```python
from build123d import *

# Parameters (mm, degrees)
LINEAR_AUSTRAGEN_D_NN1_DEPTH    = 110
SKIZZE2_R                       = 2.5
SCHNITT_LINEAR_AUSTRAGEN1_DEPTH = 17
VERRUNDUNG1_R                   = 2


with BuildPart() as part:
    # Skizze1 → Linear-Austragen-Dünn1 (new body)
    with BuildSketch(Plane.XY):
        Polygon((0, 20), (0, 0), (20, 0), (20, 1.5), (1.5, 1.5), (1.5, 20), align=None)
    extrude(amount=-LINEAR_AUSTRAGEN_D_NN1_DEPTH)

    # Skizze2 → Schnitt-Linear austragen1 (cut)
    with BuildSketch(Plane.XZ):
        with Locations(Location((6.5, -27, 0), (0, 0, 270))):
            Circle(SKIZZE2_R)
    extrude(amount=-SCHNITT_LINEAR_AUSTRAGEN1_DEPTH, mode=Mode.SUBTRACT)

    # Verrundung1
    verrundung1_edges = [part.edges().sort_by_distance(p)[0] for p in [
        (0.75, 20, -110),
        (0.75, 20, 0),
        (20, 0.75, 0),
        (20, 0.75, -110),
    ]]
    fillet(verrundung1_edges, radius=VERRUNDUNG1_R)


solid = part.part
```
For this review, take the finished solid that the model builds, in its own axes (mm). A direction names the side the tool comes from. Give positions to 0.01 mm unless a question says otherwise; leave off trailing zeros. Write each loop counter-clockwise with the first axis right and the second up, starting at its lowest first coordinate (ties: lowest second). Pieces come first, ordered by that corner, then holes. Notation, with made-up numbers: M -29.5,44.25 L -4.5,44.25 A23 cw -4.5,67.25 Z; hole C -17.75,89 d4. An arc over 180 degrees is marked long. One line per item, written item: value.
1) For P1, Ø9, axis at y = 14, z = -54, coming from the +X side, flat-tipped, find the tip position at first contact; note if it passes through.
Results are:
P1: stops at x = 1.5
2) For line 1 (X direction, y = 0.6, z = -27); line 2 (X direction, y = 10, z = -21), list the stretches that pass through material, from the lowest coordinate up. Write a range as from..to.
Results are:
line 1: x = 0..4, 9..20
line 2: x = 0..1.5
3) Take a section at C-C, the plane y = 10.25. Write out the cut boundary in (x, z), then the cut area to 3 significant figures.
Results are:
outline: M 0,-110 L 1.5,-110 L 1.5,0 L 0,0 Z
area: 165 mm²
4) Take a section at A-A, the plane z = -27. Write out the cut boundary in (x, y).
Results are:
outline: M 0,0 L 4,0 L 4,1.5 L 1.5,1.5 L 1.5,20 L 0,20 Z; M 9,0 L 20,0 L 20,1.5 L 9,1.5 Z
5) Take a section at B-B, the plane x = 6.5. Write out the cut boundary in (y, z).
Results are:
outline: M 0,-110 L 1.5,-110 L 1.5,-29.5 L 0,-29.5 Z; M 0,-24.5 L 1.5,-24.5 L 1.5,0 L 0,0 Z
6) Take a section at D-D, the plane z = -96. Write out the cut boundary in (x, y).
Results are:
outline: M 0,0 L 20,0 L 20,1.5 L 1.5,1.5 L 1.5,20 L 0,20 Z
7) For faces 1 (the cylindrical face through (0.74, 19.43, -109.4)), 2 (the flat face through (1.5, 11, -54)), list the 3-axis set-ups (+Z, -Z, +X, -X, +Y, -Y) from which the entire face can be reached by the end or side of a thin tool; tool diameter is ignored.
Results are:
face 1: -Z, +X, -X, +Y
face 2: +Z, -Z, +X, +Y
8) The part is to be moulded in two halves that separate along X. For faces 3 (the flat face through (11, 1.5, -54)), 4 (the cylindrical face through (6.6, 0.7, -24.5)), 5 (the flat face through (0, 10, -54)), say which applies: +X half, -X half, draft (parallel to the pull), parting line (faces both ways), or undercut.
Results are:
face 3: draft
face 4: undercut
face 5: -X half
